```python
from build123d import *

# Parameters (mm, degrees)
EXTRUDE_1_DEPTH          = 60
SKETCH_2_W               = 88.076446511
SKETCH_2_H               = 60
EXTRUDE_2_DEPTH          = 5
SKETCH_3_R               = 27
CUT_EXTRUDE_1_DEPTH      = 50
SKETCH_4_R               = 36.5
EXTRUDE_3_DEPTH          = 3
SKETCH_13_R              = 20
CUT_EXTRUDE_3_DEPTH      = 60
SKETCH_14_R              = 1
CUT_EXTRUDE_4_DEPTH      = 60
PATTERN_CIRCULAR_1_COUNT = 6
SKETCH_16_R              = 2
CUT_EXTRUDE_5_DEPTH      = 3
PATTERN_LINEAR_1_COUNT   = 2
PATTERN_LINEAR_1_PITCH   = 20
SKETCH_17_R              = 2
CUT_EXTRUDE_6_DEPTH      = 3
PATTERN_LINEAR_2_COUNT   = 2
PATTERN_LINEAR_2_PITCH   = 20
SKETCH_18_R              = 20
EXTRUDE_4_DEPTH          = 6
SKETCH_19_R              = 6
CUT_EXTRUDE_7_DEPTH      = 6
SKETCH_20_R              = 15
CUT_EXTRUDE_8_DEPTH      = 3
SKETCH_21_R              = 1.25
CUT_EXTRUDE_9_DEPTH      = 3
PATTERN_CIRCULAR_2_COUNT = 4


with BuildPart() as part:
    # 草图1 → 凸台-拉伸1 (new body)
    with BuildSketch(Plane.XY):
        Polygon((-67.082379863, -7.957665904), (16.917620137, -7.957665904), (16.917620137, 18.527432362), align=None)
    extrude(amount=EXTRUDE_1_DEPTH)

    # 草图2 → 凸台-拉伸2 (add)
    with BuildSketch(Plane(origin=(-3.783690806, 12.000334093, 0), x_dir=(0.9537169507482267, 0.30070579950427384, 0), z_dir=(-0.30070579950427384, 0.9537169507482267, 0))):
        with Locations((-22.332295804, -30)):
            Rectangle(SKETCH_2_W, SKETCH_2_H)
    extrude(amount=EXTRUDE_2_DEPTH)

    # 草图3 → 切除-拉伸1 (cut)
    with BuildSketch(Plane(origin=(0, -7.957665904, 0), x_dir=(-1, 0, 0), z_dir=(0, -1, 0))):
        with Locations(Location((25.082379863, -30, 0), (0, 0, 90))):
            Circle(SKETCH_3_R)
    extrude(amount=-CUT_EXTRUDE_1_DEPTH, mode=Mode.SUBTRACT)

    # 草图4 → 凸台-拉伸3 (add)
    with BuildSketch(Plane(origin=(0, -7.957665904, 0), x_dir=(-1, 0, 0), z_dir=(0, -1, 0))):
        with Locations((25.082379863, -30)):
            Circle(SKETCH_4_R)
    extrude(amount=-EXTRUDE_3_DEPTH)

    # 草图13 → 切除-拉伸3 (cut)
    with BuildSketch(Plane(origin=(0, -4.957665904, 0), x_dir=(1, 0, 0), z_dir=(0, 1, 0))):
        with Locations(Location((-25.082379863, -30, 0), (0, 0, 270))):
            Circle(SKETCH_13_R)
    extrude(amount=-CUT_EXTRUDE_3_DEPTH, mode=Mode.SUBTRACT)

    # 草图14 → 切除-拉伸4 (cut)
    with BuildSketch(Plane(origin=(0, -4.957665904, 0), x_dir=(1, 0, 0), z_dir=(0, 1, 0))):
        with Locations(Location((-48.082379863, -30, 0), (0, 0, 270))):
            Circle(SKETCH_14_R)
    cut_extrude_4 = extrude(amount=-CUT_EXTRUDE_4_DEPTH, mode=Mode.SUBTRACT)

    # 阵列(圆周)1: 切除-拉伸4 ×6 about axis
    pattern_circular_1_axis = Axis((-25.082379863, 0, 30), (0, 1, 0))
    for i in range(1, PATTERN_CIRCULAR_1_COUNT):
        add(cut_extrude_4.rotate(pattern_circular_1_axis, i * 360 / PATTERN_CIRCULAR_1_COUNT), mode=Mode.SUBTRACT)

    # 草图16 → 切除-拉伸5 (cut)
    with BuildSketch(Plane(origin=(-5.287219803, 16.768918847, 0), x_dir=(0.9537169507482267, 0.3007057995042738, 0), z_dir=(-0.3007057995042738, 0.9537169507482267, 0))):
        with Locations(Location((-61.370519059, -5, 0), (0, 0, 180))):
            Circle(SKETCH_16_R)
        with Locations(Location((-61.370519059, -55, 0), (0, 0, 180))):
            Circle(SKETCH_16_R)
    cut_extrude_5 = extrude(amount=-CUT_EXTRUDE_5_DEPTH, mode=Mode.SUBTRACT)

    # 阵列(线性)1: 切除-拉伸5 ×2
    with Locations(*[Vector(0.9537169507482268, 0.3007057995042739, 0) * (i * PATTERN_LINEAR_1_PITCH) for i in range(1, PATTERN_LINEAR_1_COUNT)]):
        add(cut_extrude_5, mode=Mode.SUBTRACT)

    # 草图17 → 切除-拉伸6 (cut)
    with BuildSketch(Plane(origin=(-5.287219803, 16.768918847, 0), x_dir=(0.9537169507482267, 0.3007057995042738, 0), z_dir=(-0.3007057995042738, 0.9537169507482267, 0))):
        with Locations(Location((16.705927452, -55, 0), (0, 0, 180))):
            Circle(SKETCH_17_R)
        with Locations(Location((16.705927452, -5, 0), (0, 0, 180))):
            Circle(SKETCH_17_R)
    cut_extrude_6 = extrude(amount=-CUT_EXTRUDE_6_DEPTH, mode=Mode.SUBTRACT)

    # 阵列(线性)2: 切除-拉伸6 ×2
    with Locations(*[Vector(-0.9537169507482268, -0.30070579950427384, 0) * (i * PATTERN_LINEAR_2_PITCH) for i in range(1, PATTERN_LINEAR_2_COUNT)]):
        add(cut_extrude_6, mode=Mode.SUBTRACT)

    # 草图18 → 凸台-拉伸4 (add)
    with BuildSketch(Plane(origin=(0, -4.957665904, 0), x_dir=(1, 0, 0), z_dir=(0, 1, 0))):
        with Locations(Location((-25.082379863, -30, 0), (0, 0, 270))):
            Circle(SKETCH_18_R)
    extrude(amount=-EXTRUDE_4_DEPTH)

    # 草图19 → 切除-拉伸7 (cut)
    with BuildSketch(Plane(origin=(0, -4.957665904, 0), x_dir=(1, 0, 0), z_dir=(0, 1, 0))):
        with Locations(Location((-25.082379863, -30, 0), (0, 0, 270))):
            Circle(SKETCH_19_R)
    extrude(amount=-CUT_EXTRUDE_7_DEPTH, mode=Mode.SUBTRACT)

    # 草图20 → 切除-拉伸8 (cut)
    with BuildSketch(Plane(origin=(0, -4.957665904, 0), x_dir=(1, 0, 0), z_dir=(0, 1, 0))):
        with Locations(Location((-25.082379863, -30, 0), (0, 0, 270))):
            Circle(SKETCH_20_R)
    extrude(amount=-CUT_EXTRUDE_8_DEPTH, mode=Mode.SUBTRACT)

    # 草图21 → 切除-拉伸9 (cut)
    with BuildSketch(Plane(origin=(0, -7.957665904, 0), x_dir=(1, 0, 0), z_dir=(0, 1, 0))):
        with Locations(Location((-33.082379863, -30, 0), (0, 0, 270))):
            Circle(SKETCH_21_R)
    cut_extrude_9 = extrude(amount=-CUT_EXTRUDE_9_DEPTH, mode=Mode.SUBTRACT)

    # 阵列(圆周)2: 切除-拉伸9 ×4 about axis
    pattern_circular_2_axis = Axis((-25.082379863, 0, 30), (0, 1, 0))
    for i in range(1, PATTERN_CIRCULAR_2_COUNT):
        add(cut_extrude_9.rotate(pattern_circular_2_axis, i * 360 / PATTERN_CIRCULAR_2_COUNT), mode=Mode.SUBTRACT)


solid = part.part
```
Geometry check sheet. Reference: the model listing, model coordinates, mm. A direction names the side the tool comes from. Give positions to 0.01 mm unless a question says otherwise; leave off trailing zeros. Order: outer loops, then holes, each group sorted by start corner. A loop starts at its lowest first (then second) coordinate and runs counter-clockwise, first axis right, second up.
1. Section check C-C, the plane x = 4. Enter the section's corners in (y, z), and give its area (3 significant figures).
2. Release check for a two-part mould opening along Y. For faces 4 (the face through (-62.89, -4.54, 55.03)), 5 (the face through (-16.604, -9.437, 28.845)), 6 (the face through (-44, -7.958, 21)) record: pulls with the +Y half, pulls with the -Y half, needs draft (parallel to the pull), parting line crosses it, or undercut.
3. Section check B-B, the plane z = 30. Give the number of separate pieces and of enclosed holes in the cut face, and give its area (3 significant figures).
4. Access from +Z, -Z, +X, -X, +Y, -Y to the whole of each face (thin tool, end or side, straight path). Record for faces 1 (the face through (-31.5, -7.958, 29.8)), 2 (the face through (11.57, 18.94, 55.03)), 3 (the face through (-49.059, -6.437, 29.783)).
5. Thickness scan on L1, parallel to X at y = -10, z = 30; L2, parallel to Z at x = -13.5, y = -6; L3, parallel to Z at x = -26, y = -1. Record the ranges inside material, lowest first.
6. Section check A-A, the plane z = 38. Enter the section's corners in (x, y).
7. Gauge pin test, flat ends, axial feed: pin 1 Ø1.5 at (x, z) = (-25.08, 38) entering from -Y; pin 2 Ø12 at (x, y) = (-22, 11) entering from -Z; pin 3 Ø12 at (y, z) = (10, 23) entering from -X; pin 4 Ø4 at (x, y) = (-32, 7.5) entering from +Z. Record the tip position at first contact, or that the pin passes through.
Values follow:
1. outline: (-7.96, 0) - (19.7, 0) - (19.7, 60) - (-7.96, 60) - close
1. area: 1,660 mm2
2. face 4: undercut
2. face 5: needs draft
2. face 6: pulls with the -Y half
3. separate pieces: 6
3. enclosed holes: 0
3. area: 684 mm2
4. face 1: +Y
4. face 2: none
4. face 3: +Y, -Y
5. L1: x = -45.08 to -34.33, -31.83 to -31.08, -19.08 to -18.33, -15.83 to -5.08
5. L2: z = -4.61 to 9.08, 11.08 to 20.47, 39.53 to 48.92, 50.92 to 64.61
5. L3: z = 0 to 3.02, 56.98 to 60
6. outline: (-68.59, -3.19) - (-67.08, -7.96) - (-43.41, -7.96) - (-43.41, -10.96) - (-26.33, -10.96) - (-26.33, -7.96) - (-37.77, -7.96) - (-37.77, -4.96) - (-50.87, -4.96) - (-50.87, 2.4) - close; (-23.83, -10.96) - (-6.75, -10.96) - (-6.75, -7.96) - (16.92, -7.96) - (16.92, 18.53) - (15.41, 23.3) - (0.71, 18.66) - (0.71, -4.96) - (-12.39, -4.96) - (-12.39, -7.96) - (-23.83, -7.96) - close
7. pin 1: passes through
7. pin 2: stops at z = 0
7. pin 3: stops at x = -1.42
7. pin 4: stops at z = 60
